The listing builds one solid part. Answer for the finished solid, in the listing's coordinates (mm). Coordinates: 2 decimals unless noted, no trailing zeros. Loops run counter-clockwise (first coordinate to the right, second up) from the corner with the lowest first, then second, coordinate; pieces in that order, holes last. Notation, with made-up numbers: M -6.5,69.5 L 46.5,69.5 A30 ccw 46.5,96.5 Z; hole C 84,-2.75 d5. An arc over 180 degrees is marked long. Answer as a JSON object with one key per item and string values. Group by question number.
1. Given pin 1 (4 mm diameter, centred on x = 14.57, y = -8.49, fed in from -Z), flat-ended and moving along its own axis, determine where the tip first touches the part or whether it passes through.
2. A cutting plane is placed at A-A on y = 20. Give the vertices of the cut face in (x, z) (3 decimals).
3. A cutting plane is placed at D-D on x = 96. Give the vertices of the cut face in (y, z) (3 decimals), and give its area (3 significant figures).
4. A cutting plane is placed at B-B on x = 0. Give the vertices of the cut face in (y, z) (3 decimals), and give its area (3 significant figures).
5. Determine the mould class of faces 1 (the face through (12.68, -9.94, 1.61)), 2 (the face through (18, -12, 0)), 3 (the face through (70.18, 0.795, 1.565)) for opening direction X: released by +X, released by -X, zero draft, split by the parting line, or undercut.
6. A cutting plane is placed at C-C on z = 2.65. State how many separate pieces and enclosed holes the cut face has, and give its area (3 significant figures).
7. Straight lines are drawn through the part: L1, parallel to Y at x = -1.5, z = 2.65; L2, parallel to Y at x = 15, z = 0.35; L3, parallel to X at y = 1, z = 2.95. For each, find the intervals that lie inside material, in ascending order.
from build123d import *

# Parameters (mm, degrees)
SKETCH1_W           = 50.8
SKETCH1_H           = 113.538
SKETCH1_R           = 14.3129
BOSS_EXTRUDE1_DEPTH = 3.175
SKETCH2_R           = 2.38125
CUT_EXTRUDE1_DEPTH  = 130.392622385
SKETCH3_R           = 2.38125
CUT_EXTRUDE2_DEPTH  = 130.392622385
SKETCH4_R           = 2.38125
CUT_EXTRUDE3_DEPTH  = 130.392622385


with BuildPart() as part:
    # Sketch1 → Boss-Extrude1 (new body)
    # profile 1 of 3: a face of its own
    with BuildSketch(Plane.XY):
        Polygon((-25.4, 56.769), (-82.181258838, -56.769), (-25.4, -56.769), align=None)
    # profile 2 of 3: a face of its own
    with BuildSketch(Plane.XY):
        Rectangle(SKETCH1_W, SKETCH1_H)
        with Locations((0, 12.319)):
            Circle(SKETCH1_R, mode=Mode.SUBTRACT)
    # profile 3 of 3: a face of its own
    with BuildSketch(Plane.XY):
        Polygon((116.231023146, -56.769), (25.4, -56.769), (25.4, 56.769), align=None)
    extrude(amount=BOSS_EXTRUDE1_DEPTH)

    # Sketch2 → Cut-Extrude1 (cut, through all)
    with BuildSketch(Plane.XY.offset(3.175)):
        with Locations((-61.630242658, -44.069)):
            Circle(SKETCH2_R)
        with Locations((-36.230242658, -44.069)):
            Circle(SKETCH2_R)
        with Locations((-50.269055108, -21.351530567)):
            Circle(SKETCH2_R)
        with Locations((-24.869055108, -21.351530567)):
            Circle(SKETCH2_R)
        with Locations((64.406974336, -44.069)):
            Circle(SKETCH2_R)
        with Locations((89.806974336, -44.069)):
            Circle(SKETCH2_R)
        with Locations((48.539653752, -24.234985342)):
            Circle(SKETCH2_R)
        with Locations((73.939653752, -24.234985342)):
            Circle(SKETCH2_R)
    extrude(amount=-CUT_EXTRUDE1_DEPTH, mode=Mode.SUBTRACT)

    # Sketch3 → Cut-Extrude2 (cut, through all)
    with BuildSketch(Plane.XY.offset(3.175)):
        with Locations((0, 44.069)):
            Circle(SKETCH3_R)
        with Locations((0, -18.669)):
            Circle(SKETCH3_R)
        with Locations((0, -44.069)):
            Circle(SKETCH3_R)
    extrude(amount=-CUT_EXTRUDE2_DEPTH, mode=Mode.SUBTRACT)

    # Sketch4 → Cut-Extrude3 (cut, through all)
    with BuildSketch(Plane.XY.offset(3.175)):
        with Locations((-14.568841483, 33.125461925)):
            Circle(SKETCH4_R)
        with Locations((14.568841483, -8.487461925)):
            Circle(SKETCH4_R)
    extrude(amount=-CUT_EXTRUDE3_DEPTH, mode=Mode.SUBTRACT)


solid = part.part
From the geometry:
{
 "1": {"pin 1": "passes through"},
 "2": {"outline": "M -43.788,0 L -12.077,0 L -12.077,3.175 L -43.788,3.175 Z; M 12.077,0 L 54.815,0 L 54.815,3.175 L 12.077,3.175 Z"},
 "3": {"outline": "M -56.769,0 L -31.48,0 L -31.48,3.175 L -56.769,3.175 Z", "area": "80.3 mm²"},
 "4": {"outline": "M -56.769,0 L -46.45,0 L -46.45,3.175 L -56.769,3.175 Z; M -41.688,0 L -21.05,0 L -21.05,3.175 L -41.688,3.175 Z; M -16.288,0 L -1.994,0 L -1.994,3.175 L -16.288,3.175 Z; M 26.632,0 L 41.688,0 L 41.688,3.175 L 26.632,3.175 Z; M 46.45,0 L 56.769,0 L 56.769,3.175 L 46.45,3.175 Z", "area": "224 mm²"},
 "5": {"face 1": "undercut", "face 2": "zero draft", "face 3": "released by +X"},
 "6": {"separate pieces": "1", "enclosed holes": "14", "area": "13,300 mm²"},
 "7": {"L1": "y = -56.77 to -45.92, -42.22 to -20.52, -16.82 to -1.92, 26.55 to 42.22, 45.92 to 56.77", "L2": "y = -56.77 to -10.83, -6.15 to 56.77", "L3": "x = -53.29 to -8.76, 8.76 to 70.02"}
}
